Geometry: final body of the model. Coordinates: model frame, mm. Face numbers are marked on the shaded views. A direction names the side the tool comes from. Coordinates: 2 decimals unless noted, no trailing zeros. Order: outer loops, then holes, each group sorted by start corner. A loop starts at its lowest first (then second) coordinate and runs counter-clockwise, first axis right, second up. Notation, with made-up numbers: M -31.75,1.25 L 15.25,1.25 A17 cw 15.25,9.25 Z; hole C -20.75,57 d10. An arc over 180 degrees is marked long. Write item = value, one per line.
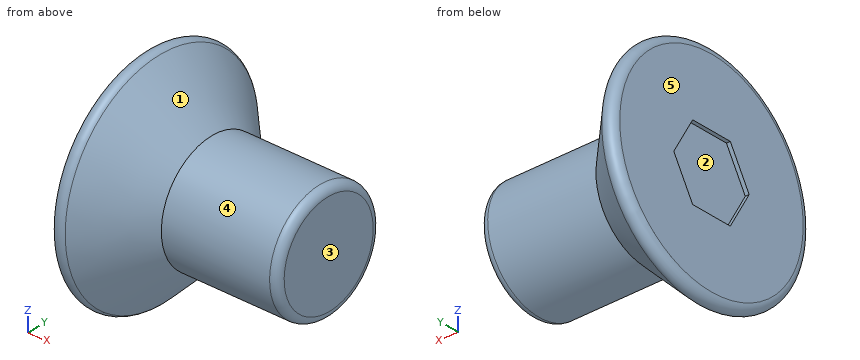
from build123d import *

# Parameters (mm, degrees)
ENL_V_MAT_EXTRU_1_DEPTH = 0.1
CONG_1_R                = 0.2


with BuildPart() as part:
    # Esquisse1 → Révolution1 (revolve)
    with BuildSketch(Plane.XY, mode=Mode.PRIVATE) as r_volution1_sk:
        Polygon((0, 0), (0, 3.16), (1.66, 1.5), (4.66, 1.5), (4.66, 0), align=None)
    revolve(r_volution1_sk.sketch.rotate(Axis((-5.768945874, 0, 0), (1, 0, 0)), 90), axis=Axis((-5.768945874, 0, 0), (1, 0, 0)))

    # Esquisse2 → Enlèv. mat.-Extru.1 (cut)
    with BuildSketch(Plane.ZY):
        Polygon((0, -1.1), (0.952627944, -0.55), (0.952627944, 0.55), (0, 1.1), (-0.952627944, 0.55), (-0.952627944, -0.55), align=None)
    extrude(amount=-ENL_V_MAT_EXTRU_1_DEPTH, mode=Mode.SUBTRACT)

    # Congé1
    cong_1_edges = [part.edges().sort_by_distance(p)[0] for p in [
        (4.66, 0, -1.5),
        (0, 0, -3.16),
    ]]
    fillet(cong_1_edges, radius=CONG_1_R)


solid = part.part
1) Pin query (flat end, axial travel): pin 1 (1.5 mm diameter, centred on x = 2.5, y = 2, fed in from +Z); pin 2 (1.5 mm diameter, centred on x = 1, y = -2, fed in from -Z). Return the tip coordinate at first contact, or that it passes through.
Numbers:
pin_1 = 0.83
pin_2 = -2.29
2) Mould query, pull axis Y, two halves, no side actions, for the marked faces 1, 2 and 3. Classes: pulls with the +Y half, pulls with the -Y half, needs draft (parallel to the pull), parting line crosses it, or undercut.
Numbers:
face_1 = parting line crosses it
face_2 = undercut
face_3 = needs draft
3) Section A-A, the plane y = 0. Return loops of the section in (x, z).
Numbers:
outline = M 0,-2.68 A0.2 ccw 0.34,-2.82 L 1.66,-1.5 L 4.46,-1.5 A0.2 ccw 4.66,-1.3 L 4.66,1.3 A0.2 ccw 4.46,1.5 L 1.66,1.5 L 0.34,2.82 A0.2 ccw 0,2.68 L 0,0.95 L 0.1,0.95 L 0.1,-0.95 L 0,-0.95 Z
4) Set-up query: the marked faces 4 and 5. Return all of +Z, -Z, +X, -X, +Y, -Y with unobstructed straight access to the full face (end or side cutting, diameter ignored); none if empty.
Numbers:
face_4 = +X
face_5 = +Z, -Z, -X, +Y, -Y
5) Line query: L1, parallel to Y at x = 2.7, z = 0; L2, parallel to X at y = -2.05, z = 1.2; L3, parallel to Z at x = 4.05, y = -0.75. Output: solid intervals per line, ascending.
Numbers:
L1 = -1.5 to 1.5
L2 = 0 to 0.78
L3 = -1.3 to 1.3
6) Section B-B, the plane x = 4.3. Return loops of the section in (y, z).
Numbers:
outline = C 0,0 d3
